```python
from build123d import *

# Parameters (mm, degrees)
SKETCH1_R           = 2.286
BOSS_EXTRUDE1_DEPTH = 3.96875


with BuildPart() as part:
    # Sketch1 → Boss-Extrude1 (new, symmetric)
    with BuildSketch(Plane.XY):
        with BuildLine():
            Line((55.852160303, 20.499543888), (12.426339018, 21.289226167))
            ThreePointArc((12.426339018, 21.289226167), (0.183355577, 16.585853064), (-5.332604413, 4.686838505))
            Line((-5.332604413, 4.686838505), (-5.549551288, 0.272753664))
            ThreePointArc((-5.549551288, 0.272753664), (-0.272753664, -5.549551288), (5.549551288, -0.272753664))
            Line((5.549551288, -0.272753664), (5.766498164, 4.141331178))
            ThreePointArc((5.766498164, 4.141331178), (7.688680768, 8.388633469), (11.993389211, 10.178563055))
            Line((11.993389211, 10.178563055), (17.405800458, 10.276985724))
            ThreePointArc((17.405800458, 10.276985724), (26.626022332, 8.622204767), (34.517045693, 3.574181217))
            ThreePointArc((34.517045693, 3.574181217), (36.773296982, 2.690364107), (38.995923428, 3.65562793))
            ThreePointArc((38.995923428, 3.65562793), (46.698197557, 8.987209748), (55.852160303, 10.976118364))
            ThreePointArc((55.852160303, 10.976118364), (60.528070342, 15.737831126), (55.852160303, 20.499543888))
        make_face()
        Circle(SKETCH1_R, mode=Mode.SUBTRACT)
        with Locations((55.765570342, 15.737831126)):
            Circle(SKETCH1_R, mode=Mode.SUBTRACT)
    extrude(amount=BOSS_EXTRUDE1_DEPTH, both=True)


solid = part.part
```
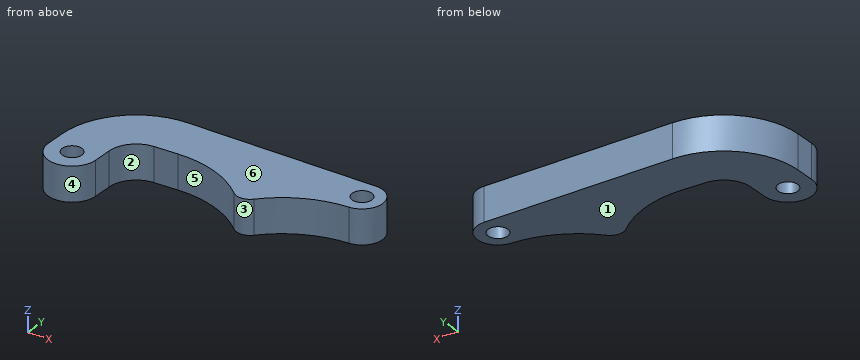
Design review of the part built by this model. Coordinates are the model's own, in mm. Face numbers are marked on the shaded views. A direction names the side the tool comes from. Give positions to 0.01 mm unless a question says otherwise; leave off trailing zeros. Order: outer loops, then holes, each group sorted by start corner. A loop starts at its lowest first (then second) coordinate and runs counter-clockwise, first axis right, second up. Notation, with made-up numbers: (88.5, 64) -> (137.5, 64) arc R22 cw to (137.5, 103) -> close; hole circle Ø1 at (-26, 88.25). An arc over 180 degrees is marked (long way). Write item = value, one per line. Start each with the question number.
(1) For pin 1 (12 mm diameter, centred on x = 31.5, y = -2, fed in from -Z); pin 2 (1 mm diameter, centred on x = 41, z = 2, fed in from -Y); pin 3 (1 mm diameter, centred on y = 3.5, z = 0, fed in from +X), all flat-tipped, find the tip position at first contact; note any pin that passes through.
(2) Mouldability with a two-part tool opening along X and no side actions: class the marked faces 1, 2, 3 and 4 as +X half, -X half, draft (parallel to the pull), parting line (faces both ways), or undercut.
(3) We need section C-C on z = 3. State how many separate pieces and enclosed holes the cut face has, plus the area to 3 significant figures.
(4) To check wall thickness, follow line 1 along X through (y, z) = (6, -2); line 2 along X through (y, z) = (-2, 2); line 3 along Y through (x, z) = (25.5, -2.5). State the ranges of each line that lie inside material, in increasing order.
(5) We need section B-B on y = 7. Write out the cut boundary in (x, z), plus the area to 3 significant figures.
(6) We need section A-A on x = 0. Write out the cut boundary in (y, z), plus the area to 3 significant figures.
(7) We need section D-D on x = 49.5. Write out the cut boundary in (y, z).
(8) For the marked faces 5 and 6, list the 3-axis set-ups (+Z, -Z, +X, -X, +Y, -Y) from which the entire face can be reached by the end or side of a thin tool; tool diameter is ignored.
Numbers:
q1.pin_1 = through
q1.pin_2 = 5.08
q1.pin_3 = 39.34
q2.face_1 = draft
q2.face_2 = undercut
q2.face_3 = undercut
q2.face_4 = parting line
q3.separate_pieces = 1
q3.enclosed_holes = 2
q3.area = 861 mm^2
q4.line_1 = -5.22 to 6.14, 31.55 to 41.63
q4.line_2 = -5.18 to -1.11, 1.11 to 5.18
q4.line_3 = 9.03 to 21.05
q5.outline = (-5.06, -3.97) -> (6.61, -3.97) -> (6.61, 3.97) -> (-5.06, 3.97) -> close; (29.98, -3.97) -> (43.03, -3.97) -> (43.03, 3.97) -> (29.98, 3.97) -> close
q5.area = 196 mm^2
q6.outline = (-5.56, -3.97) -> (-2.29, -3.97) -> (-2.29, 3.97) -> (-5.56, 3.97) -> close; (2.29, -3.97) -> (16.41, -3.97) -> (16.41, 3.97) -> (2.29, 3.97) -> close
q6.area = 138 mm^2
q7.outline = (10, -3.97) -> (20.62, -3.97) -> (20.62, 3.97) -> (10, 3.97) -> close
q8.face_5 = +Z, -Z, -Y
q8.face_6 = +Z, +X, -X, +Y, -Y
